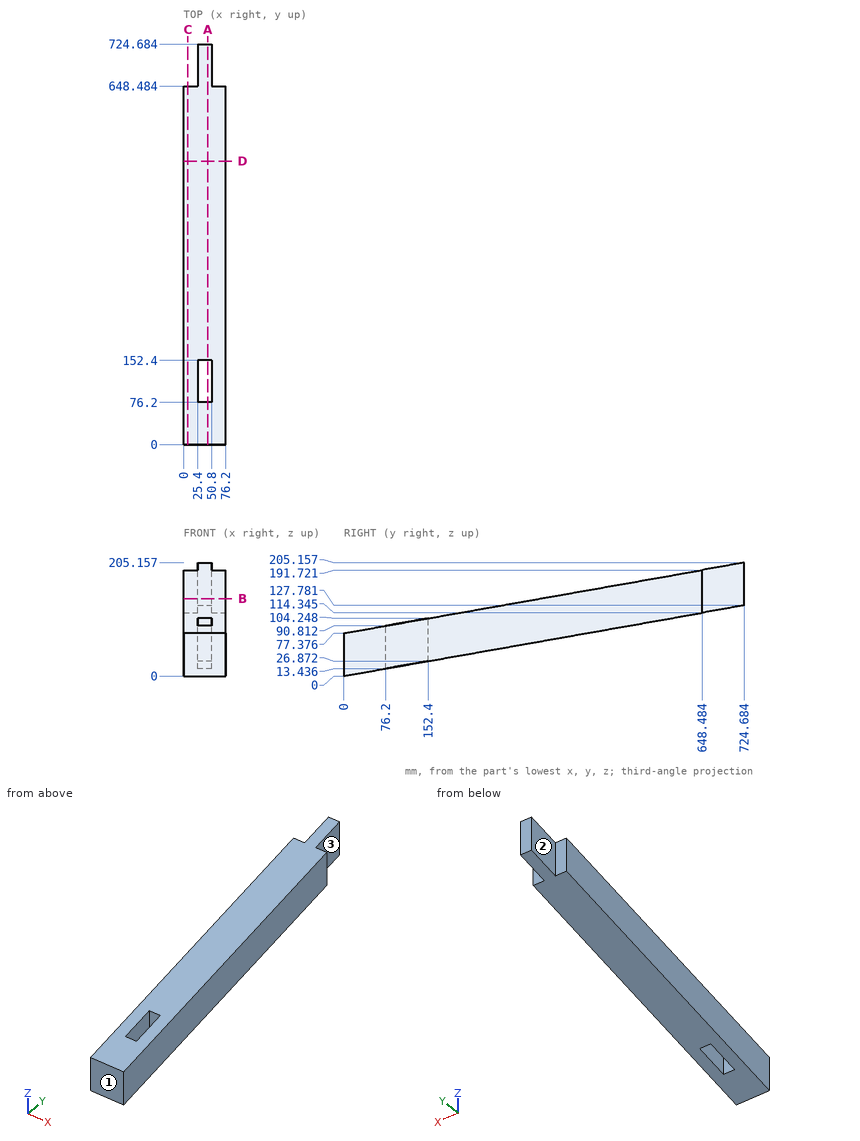
Verification items for this drawing (mm, ordinates from the low corner). A direction names the side the tool comes from. Give positions to 0.01 mm unless a question says otherwise; leave off trailing zeros. Order: outer loops, then holes, each group sorted by start corner. A loop starts at its lowest first (then second) coordinate and runs counter-clockwise, first axis right, second up. Notation, with made-up numbers: M 4.5,84 L 25.5,84 A31 ccw 25.5,120 Z; hole C 24.25,47.5 d8. An arc over 180 degrees is marked long. Use a Markdown table: item, result.
Item 1: Material ranges on line 1 along X through (y, z) = (93.5, 74.5); line 2 along Z through (x, y) = (66, 399.5); line 3 along Z through (x, y) = (13, 134.5) (1 decimal), recorded low to high.
Answers follow:
| item | result |
|---|---|
| line 1 | x = 0 to 25.4, 50.8 to 76.2 |
| line 2 | z = 70.44 to 147.82 |
| line 3 | z = 23.7 to 101.1 |
Item 2: Section check C-C (x = 7.5). Record the cut outline in (y, z) (1 decimal).
Answers follow:
| item | result |
|---|---|
| outline | M 0,0 L 648.5,114.3 L 648.5,191.7 L 0,77.4 Z |
Item 3: Section check D-D (y = 513). Record the cut outline in (x, z) (1 decimal).
Answers follow:
| item | result |
|---|---|
| outline | M 0,90.5 L 76.2,90.5 L 76.2,167.8 L 0,167.8 Z |
Item 4: Depth check by flat-ended pin: P1, Ø1, axis at x = 36.5, y = 457.5, coming from the +Z side; P2, Ø1.5, axis at x = 16.5, y = 351.5, coming from the +Z side; P3, Ø5, axis at x = 13.5, z = 176.5, coming from the +Y side. Enter the tip coordinate at first touch or a pass-through.
Answers follow:
| item | result |
|---|---|
| P1 | stops at z = 158.13 |
| P2 | stops at z = 139.49 |
| P3 | stops at y = 648.48 |
Item 5: Section check B-B (z = 140). Record the cut outline in (x, y) (1 decimal), and give its area (3 significant figures).
Answers follow:
| item | result |
|---|---|
| outline | M 0,355.2 L 76.2,355.2 L 76.2,648.5 L 50.8,648.5 L 50.8,724.7 L 25.4,724.7 L 25.4,648.5 L 0,648.5 Z |
| area | 24,300 mm2 |
Item 6: Tool access check on the marked faces 1, 2 and 3. Record the directions out of +Z, -Z, +X, -X, +Y, -Y that give a thin tool (end or side, any length) a straight path to the whole face; none if there is none.
Answers follow:
| item | result |
|---|---|
| face 1 | +Z, -Z, +X, -X, -Y |
| face 2 | +Z, -Z, -X, +Y |
| face 3 | +Z, -Z, +X, +Y |
Item 7: Section check A-A (x = 44). Record the cut outline in (y, z) (1 decimal), and give its area (3 significant figures).
Answers follow:
| item | result |
|---|---|
| outline | M 0,0 L 76.2,13.4 L 76.2,90.8 L 0,77.4 Z; M 152.4,26.9 L 724.7,127.8 L 724.7,205.2 L 152.4,104.2 Z |
| area | 50,200 mm2 |
